Could you check a few things on this drawing? It's one solid part, dimensions in mm from its lowest x, y, z. Coordinates: 2 decimals unless noted, no trailing zeros. Write each loop counter-clockwise with the first axis right and the second up, starting at its lowest first coordinate (ties: lowest second). Pieces come first, ordered by that corner, then holes. Notation, with made-up numbers: (-7.5, 5.5) - (45.5, 5.5) arc R5 ccw to (45.5, 10.5) - close; hole circle Ø3 at (53, -2.75). An arc over 180 degrees is marked (long way). Write each question's results on one line, items separated by ' | '. Start each with the question number.
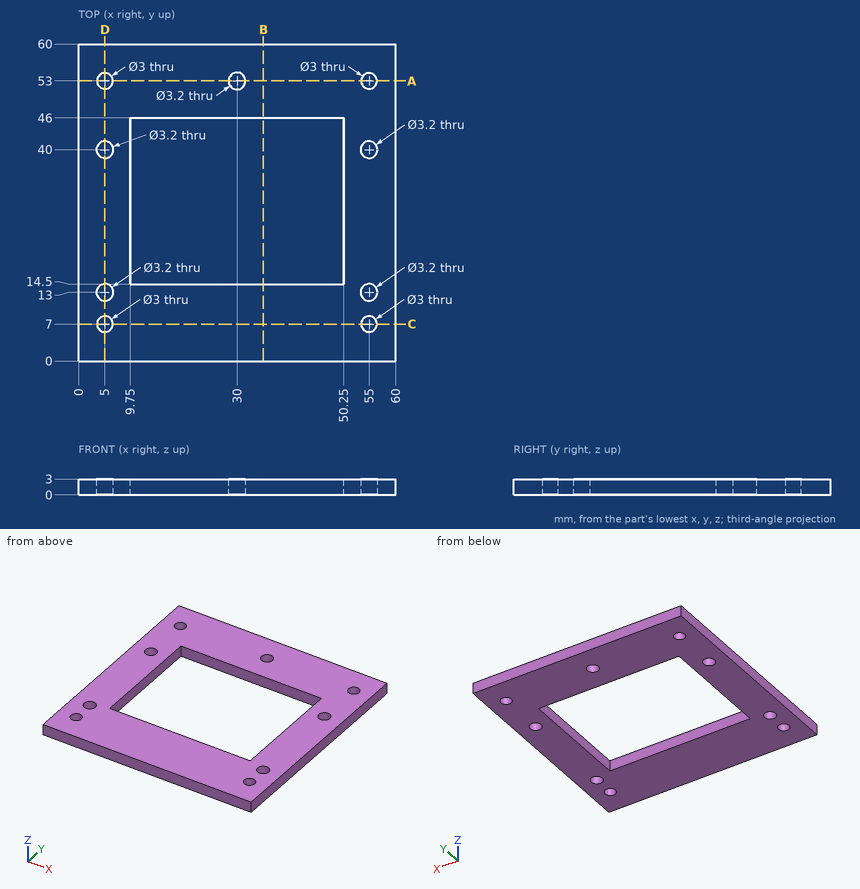
Q1. If we section it at B-B (x = 35): Please give me the cut outline in (y, z).
Q2. If we section it at A-A (y = 53): Please give me the cut outline in (x, z), then the cut area to 3 significant figures.
Q3. If we section it at D-D (x = 5): Please give me the cut outline in (y, z), then the cut area to 3 significant figures.
Q4. If we section it at C-C (y = 7): Please give me the cut outline in (x, z), then the cut area to 3 significant figures.
Q5. I need wall thicknesses on line 1 along Y through (x, z) = (55, 2.3); line 2 along Y through (x, z) = (30, 1.45); line 3 along X through (y, z) = (42.5, 2.1). Which ranges of each line are inside material? Lowest first, please. Write a range as from..to.
Answer list:
1) outline: (0, 0) - (14.5, 0) - (14.5, 3) - (0, 3) - close; (46, 0) - (60, 0) - (60, 3) - (46, 3) - close
2) outline: (0, 0) - (3.5, 0) - (3.5, 3) - (0, 3) - close; (6.5, 0) - (28.4, 0) - (28.4, 3) - (6.5, 3) - close; (31.6, 0) - (53.5, 0) - (53.5, 3) - (31.6, 3) - close; (56.5, 0) - (60, 0) - (60, 3) - (56.5, 3) - close | area: 152 mm2
3) outline: (0, 0) - (5.5, 0) - (5.5, 3) - (0, 3) - close; (8.5, 0) - (11.4, 0) - (11.4, 3) - (8.5, 3) - close; (14.6, 0) - (38.4, 0) - (38.4, 3) - (14.6, 3) - close; (41.6, 0) - (51.5, 0) - (51.5, 3) - (41.6, 3) - close; (54.5, 0) - (60, 0) - (60, 3) - (54.5, 3) - close | area: 143 mm2
4) outline: (0, 0) - (3.5, 0) - (3.5, 3) - (0, 3) - close; (6.5, 0) - (53.5, 0) - (53.5, 3) - (6.5, 3) - close; (56.5, 0) - (60, 0) - (60, 3) - (56.5, 3) - close | area: 162 mm2
5) line 1: y = 0..5.5, 8.5..11.4, 14.6..38.4, 41.6..51.5, 54.5..60 | line 2: y = 0..14.5, 46..51.4, 54.6..60 | line 3: x = 0..9.75, 50.25..60
